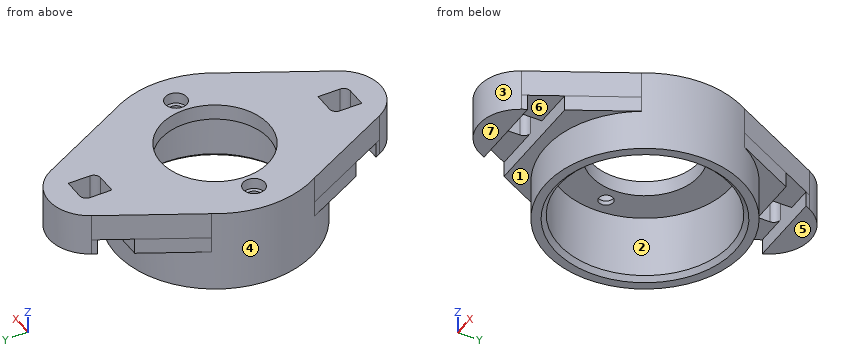
from build123d import *

# Parameters (mm, degrees)
SKETCH1_R           = 22.3
SKETCH1_R_2         = 19.3
SKETCH1_R_3         = 1.6
SKETCH1_R_4         = 12.155
BOSS_EXTRUDE1_DEPTH = 1
BOSS_EXTRUDE2_START = -15.2
SKETCH1_3_R         = 22.3
SKETCH1_3_R_2       = 19.3
BOSS_EXTRUDE2_DEPTH = 15.2
SKETCH3_R           = 22.3
SKETCH3_R_2         = 2.425
SKETCH3_R_3         = 12.155
BOSS_EXTRUDE3_DEPTH = 2.5
BOSS_EXTRUDE4_START = -6
SKETCH4_W           = 6
SKETCH4_H           = 6.4
BOSS_EXTRUDE4_DEPTH = 6
CHAMFER1_SIZE       = 1
BOSS_EXTRUDE5_START = 3.5
BOSS_EXTRUDE5_DEPTH = 3.5
FILLET1_R           = 1.5


with BuildPart() as part:
    # Sketch1 → Boss-Extrude1 (new body)
    # profile 1 of 2: a face of its own
    with BuildSketch(Plane.XY):
        Circle(SKETCH1_R)
        Circle(SKETCH1_R_2, mode=Mode.SUBTRACT)
    # profile 2 of 2: a face of its own
    with BuildSketch(Plane.XY):
        Circle(SKETCH1_R_2)
        with Locations((15.5275, 0)):
            Circle(SKETCH1_R_3, mode=Mode.SUBTRACT)
        with Locations((-15.5275, 0)):
            Circle(SKETCH1_R_3, mode=Mode.SUBTRACT)
        Circle(SKETCH1_R_4, mode=Mode.SUBTRACT)
    extrude(amount=BOSS_EXTRUDE1_DEPTH)

    # Sketch1_3 → Boss-Extrude2 (add)
    with BuildSketch(Plane.XY.offset(BOSS_EXTRUDE2_START)):
        Circle(SKETCH1_3_R)
        Circle(SKETCH1_3_R_2, mode=Mode.SUBTRACT)
    extrude(amount=BOSS_EXTRUDE2_DEPTH)

    # Sketch3 → Boss-Extrude3 (add)
    with BuildSketch(Plane.XY.offset(1)):
        Circle(SKETCH3_R)
        with Locations((-15.5275, 0)):
            Circle(SKETCH3_R_2, mode=Mode.SUBTRACT)
        with Locations((15.5275, 0)):
            Circle(SKETCH3_R_2, mode=Mode.SUBTRACT)
        Circle(SKETCH3_R_3, mode=Mode.SUBTRACT)
    extrude(amount=BOSS_EXTRUDE3_DEPTH)

    # Sketch4 → Boss-Extrude4 (add)
    # profile 1 of 2: a face of its own
    with BuildSketch(Plane.XY.offset(3.5).offset(BOSS_EXTRUDE4_START)):
        with BuildLine():
            ThreePointArc((19.110610408, -11.49237007), (0, -22.3), (-19.110610408, -11.49237007))
            Line((-19.110610408, -11.49237007), (-8.137060123, -32.292814061))
            ThreePointArc((-8.137060123, -32.292814061), (0, -37.2), (8.137060123, -32.292814061))
            Line((8.137060123, -32.292814061), (19.110610408, -11.49237007))
        make_face()
        with Locations((0, -28)):
            Rectangle(SKETCH4_W, SKETCH4_H, mode=Mode.SUBTRACT)
    # profile 2 of 2: a face of its own
    with BuildSketch(Plane.XY.offset(3.5).offset(BOSS_EXTRUDE4_START)):
        with BuildLine():
            Line((-8.137060123, 32.292814061), (-19.110610408, 11.49237007))
            ThreePointArc((-19.110610408, 11.49237007), (0, 22.3), (19.110610408, 11.49237007))
            Line((19.110610408, 11.49237007), (8.137060123, 32.292814061))
            ThreePointArc((8.137060123, 32.292814061), (0, 37.2), (-8.137060123, 32.292814061))
        make_face()
        with Locations((0, 28)):
            Rectangle(SKETCH4_W, SKETCH4_H, mode=Mode.SUBTRACT)
    extrude(amount=BOSS_EXTRUDE4_DEPTH)

    # Chamfer1
    chamfer1_edges = [part.edges().sort_by_distance(p)[0] for p in [
        (-19.3, 0, -15.2),
    ]]
    chamfer(chamfer1_edges, length=CHAMFER1_SIZE)

    # Sketch5 → Boss-Extrude5 (add)
    with BuildSketch(Plane(origin=(0, 0, -2.5), x_dir=(-1, 0, 0), z_dir=(0, 0, -1)).offset(BOSS_EXTRUDE5_START)):
        with BuildLine():
            Line((12.089993623, 24.8), (-12.089993623, 24.8))
            Line((-12.089993623, 24.8), (-19.110610408, 11.49237007))
            ThreePointArc((-19.110610408, 11.49237007), (0, 22.3), (19.110610408, 11.49237007))
            Line((19.110610408, 11.49237007), (12.089993623, 24.8))
        make_face()
        with BuildLine():
            ThreePointArc((8.137060123, 32.292814061), (0, 37.2), (-8.137060123, 32.292814061))
            Line((-8.137060123, 32.292814061), (-8.713588684, 31.2))
            Line((-8.713588684, 31.2), (8.713588684, 31.2))
            Line((8.713588684, 31.2), (8.137060123, 32.292814061))
        make_face()
        with BuildLine():
            Line((-19.110610408, -11.49237007), (-12.089993623, -24.8))
            Line((-12.089993623, -24.8), (12.089993623, -24.8))
            Line((12.089993623, -24.8), (19.110610408, -11.49237007))
            ThreePointArc((19.110610408, -11.49237007), (0, -22.3), (-19.110610408, -11.49237007))
        make_face()
        with BuildLine():
            Line((8.713588684, -31.2), (-8.713588684, -31.2))
            Line((-8.713588684, -31.2), (-8.137060123, -32.292814061))
            ThreePointArc((-8.137060123, -32.292814061), (0, -37.2), (8.137060123, -32.292814061))
            Line((8.137060123, -32.292814061), (8.713588684, -31.2))
        make_face()
    extrude(amount=-BOSS_EXTRUDE5_DEPTH)

    # Fillet1
    fillet1_edges = [part.edges().sort_by_distance(p)[0] for p in [
        (-3, 31.2, 0.5),
        (3, 24.8, 0.5),
        (3, -31.2, 0.5),
        (-3, -24.8, 0.5),
    ]]
    fillet(fillet1_edges, radius=FILLET1_R)


solid = part.part
The listing builds one solid part. Answer for the finished solid, in the listing's coordinates (mm). Face numbers are marked on the shaded views. A direction names the side the tool comes from. Round coordinates to 2 decimals unless told otherwise and drop trailing zeros. Write each loop counter-clockwise with the first axis right and the second up, starting at its lowest first coordinate (ties: lowest second). Pieces come first, ordered by that corner, then holes. Notation, with made-up numbers: M -33.75,53.5 L 13.25,53.5 A17 cw 13.25,63.5 Z; hole C 61,49.5 d4. An arc over 180 degrees is marked long. Write each question's results on one line, items separated by ' | '. Start each with the question number.
Item 1: Straight lines are drawn through the part: probe 1 along Y at (x, z) = (0, 1.8) (3 decimals); probe 2 along Y at (x, z) = (0, -3); probe 3 along Y at (x, z) = (13, -4.75) (3 decimals). For each, find the intervals that lie inside material, in ascending order.
Item 2: Find section A-A on x = 0. Write down the section's boundary in (y, z) (3 decimals).
Item 3: The mould has two halves that part along Y. Classify the marked faces 1, 2 and 3: +Y half, -Y half, draft (parallel to the pull), parting line (faces both ways), or undercut.
Item 4: Find section C-C on z = -9. Write down the section's boundary in (x, y).
Item 5: Given pin 1 Ø6 at (x, y) = (12.5, 7) entering from -Z; pin 2 Ø6 at (y, z) = (-18, -11.5) entering from +X; pin 3 Ø5 at (x, y) = (4.5, 28) entering from -Z, each flat-ended and moving along its own axis, determine where each tip first touches the part or whether it passes through.
Item 6: Find section B-B on y = 0. Give the number of separate pieces and of enclosed holes in the cut face, and give its area (3 significant figures).
Item 7: Which of the six approach directions +Z, -Z, +X, -X, +Y, -Y give full straight-line access (tool end or side, diameter ignored) to the marked faces 4, 5, 6 and 7?
Answer block:
1) probe 1: y = -37.2 to -31.2, -24.8 to -12.155, 12.155 to 24.8, 31.2 to 37.2 | probe 2: y = -37.2 to -31.2, -24.8 to -19.3, 19.3 to 24.8, 31.2 to 37.2 | probe 3: y = -23.075 to -14.265, 14.265 to 23.075
2) outline: M -37.2,-6 L -31.2,-6 L -31.2,3.5 L -37.2,3.5 Z; M -24.8,-6 L -22.3,-6 L -22.3,-15.2 L -20.3,-15.2 L -19.3,-14.2 L -19.3,0 L -12.155,0 L -12.155,3.5 L -24.8,3.5 Z; M 12.155,0 L 19.3,0 L 19.3,-14.2 L 20.3,-15.2 L 22.3,-15.2 L 22.3,-6 L 24.8,-6 L 24.8,3.5 L 12.155,3.5 Z; M 31.2,-6 L 37.2,-6 L 37.2,3.5 L 31.2,3.5 Z
3) face 1: draft | face 2: undercut | face 3: -Y half
4) outline: C 0,0 d44.6; hole C 0,0 d38.6
5) pin 1: stops at z = 0 | pin 2: stops at x = 16.5 | pin 3: stops at z = -2.5
6) separate pieces: 4 | enclosed holes: 0 | area: 131 mm²
7) face 4: -Z | face 5: -Z, +X, -X, +Y | face 6: -Z, +X, -X | face 7: -Z, +X, -X, -Y
